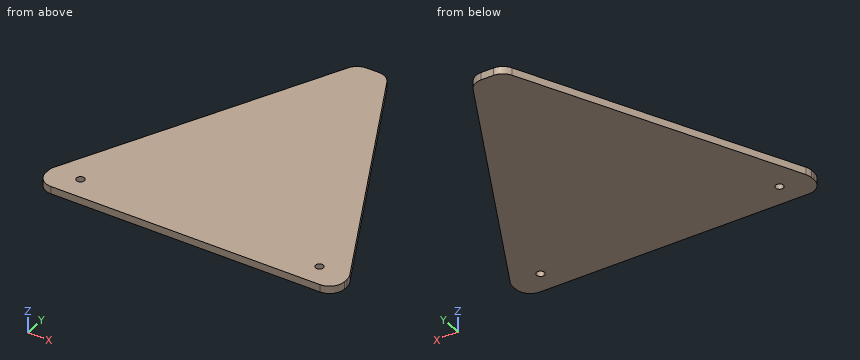
from build123d import *

# Parameters (mm, degrees)
SKETCH1_R           = 3.3734375
BOSS_EXTRUDE1_DEPTH = 6.35
FILLET2_R           = 12.7


with BuildPart() as part:
    # Sketch1 → Boss-Extrude1 (new body)
    with BuildSketch(Plane.XY):
        Polygon((0, 0), (254, 0), (254, 19.05), (140.024244399, 247.65), (113.975755601, 247.65), (0, 19.05), align=None)
        with Locations((25.4, 19.05)):
            Circle(SKETCH1_R, mode=Mode.SUBTRACT)
        with Locations((228.6, 19.05)):
            Circle(SKETCH1_R, mode=Mode.SUBTRACT)
    extrude(amount=BOSS_EXTRUDE1_DEPTH)

    # Fillet2
    fillet2_edges = [part.edges().sort_by_distance(p)[0] for p in [
        (0, 19.05, 3.175),
        (113.975755601, 247.65, 3.175),
        (140.024244399, 247.65, 3.175),
        (254, 19.05, 3.175),
        (254, 0, 3.175),
        (0, 0, 3.175),
    ]]
    fillet(fillet2_edges, radius=FILLET2_R)


solid = part.part
Geometry check sheet. Reference: the model listing, model coordinates, mm. Round coordinates to 2 decimals unless told otherwise and drop trailing zeros. Loops run counter-clockwise (first coordinate to the right, second up) from the corner with the lowest first, then second, coordinate; pieces in that order, holes last.
Item 1: Cross-section at A-A on z = 1. Record the boundary of the cut face in (x, y).
Item 2: Cross-section at B-B on x = 25.4. Record the boundary of the cut face in (y, z).
Item 3: Gauge pin test, flat ends, axial feed: pin 1 (1.5 mm diameter, centred on x = 163.5, z = 2, fed in from +Y); pin 2 (1.5 mm diameter, centred on y = 168, z = 1.5, fed in from -X). Record the tip position at first contact, or that the pin passes through.
Item 4: Cross-section at C-C on y = 193.5. Record the boundary of the cut face in (x, z).
Item 5: Cross-section at D-D on x = 89. Record the boundary of the cut face in (y, z), then the cut area to 3 significant figures.
Item 6: Thickness scan on line 1 (X direction, y = 16.5, z = 4.5); line 2 (Y direction, x = 25.4, z = 3.5); line 3 (Y direction, x = 27.5, z = 1.25). Record the ranges inside material, lowest first.
Answer sheet:
1. outline: (0, 12.7) arc R12.7 ccw to (12.7, 0) - (241.3, 0) arc R12.7 ccw to (254, 12.7) - (254, 16.06) arc R12.7 ccw to (252.67, 21.73) - (143.53, 240.62) arc R12.7 ccw to (132.17, 247.65) - (121.83, 247.65) arc R12.7 ccw to (110.47, 240.62) - (1.33, 21.73) arc R12.7 ccw to (0, 16.06) - close; hole circle Ø6.75 at (25.4, 19.05); hole circle Ø6.75 at (228.6, 19.05)
2. outline: (0, 0) - (15.68, 0) - (15.68, 6.35) - (0, 6.35) - close; (22.42, 0) - (69.99, 0) - (69.99, 6.35) - (22.42, 6.35) - close
3. pin 1: stops at y = 202.07
3. pin 2: stops at x = 73.89
4. outline: (86.98, 0) - (167.02, 0) - (167.02, 6.35) - (86.98, 6.35) - close
5. outline: (0, 0) - (197.56, 0) - (197.56, 6.35) - (0, 6.35) - close
5. area: 1,250 mm2
6. line 1: x = 0.01 to 23.19, 27.61 to 226.39, 230.81 to 253.99
6. line 2: y = 0 to 15.68, 22.42 to 69.99
6. line 3: y = 0 to 16.41, 21.69 to 74.21
